Model file for the job. Use its own axes, mm. A direction names the side the tool comes from. Give positions to 0.01 mm unless a question says otherwise; leave off trailing zeros. Loops run counter-clockwise (first coordinate to the right, second up) from the corner with the lowest first, then second, coordinate; pieces in that order, holes last. Notation, with made-up numbers: M 33.5,27 L 37.5,27 A27 cw 37.5,59 Z; hole C -26,57 d10. An arc over 180 degrees is marked long. Answer in a Markdown table with one row per item.
```python
from build123d import *

# Parameters (mm, degrees)
SKETCH2_OUTSIDE_W       = 34.798
SKETCH2_OUTSIDE_H       = 34.798
CUT_EXTRUDE1_DEPTH      = 21.32
CUT_EXTRUDE1_DEPTH_BACK = 27.67
SKETCH3_R               = 5.55625
CUT_EXTRUDE2_DEPTH      = 20.05


with BuildPart() as part:
    # Sketch1 → Revolve1 (revolve)
    with BuildSketch(Plane.XY):
        Polygon((0, 10.795), (-7.62, 10.795), (-7.62, 7.747), (-27.94, 7.747), (-27.94, 0), (19.05, 0), (19.05, 5.55625), (0, 5.55625), align=None)
    revolve(axis=Axis((-27.94, 0, 0), (1, 0, 0)))

    # Sketch2 outside → Cut-Extrude1 (cut, two sides)
    with BuildSketch(Plane.ZY.offset(7.62)) as cut_extrude1_sk:
        Rectangle(SKETCH2_OUTSIDE_W, SKETCH2_OUTSIDE_H)
        Polygon((-5.499261314, 9.525), (-10.998522628, 0), (-5.499261314, -9.525), (5.499261314, -9.525), (10.998522628, 0), (5.499261314, 9.525), align=None, mode=Mode.SUBTRACT)
    extrude(amount=CUT_EXTRUDE1_DEPTH, mode=Mode.SUBTRACT)
    extrude(cut_extrude1_sk.sketch, amount=-CUT_EXTRUDE1_DEPTH_BACK, mode=Mode.SUBTRACT)

    # Sketch3 → Cut-Extrude2 (cut, through all)
    with BuildSketch(Plane(origin=(0, 0, 0), x_dir=(0, 0, -1), z_dir=(1, 0, 0))):
        Circle(SKETCH3_R)
    extrude(amount=CUT_EXTRUDE2_DEPTH, mode=Mode.SUBTRACT)


solid = part.part
```
Q1. Saw through at A-A (x = -4.5). Give the cut face in (y, z) (3 decimals), and give its area (3 significant figures).
Reported:
| item | result |
|---|---|
| outline | M -9.525,-5.08 A10.795 ccw -9.162,-5.709 L -0.363,-10.789 A10.795 ccw 0.363,-10.789 L 9.162,-5.709 A10.795 ccw 9.525,-5.08 L 9.525,5.08 A10.795 ccw 9.162,5.709 L 0.363,10.789 A10.795 ccw -0.363,10.789 L -9.162,5.709 A10.795 ccw -9.525,5.08 Z |
| area | 314 mm² |
Q2. Probe probe 1 along X at (y, z) = (7.25, 4); probe 2 along Z at (x, y) = (-5.25, 4); probe 3 along Y at (x, z) = (-9.5, 0.5). List the from-to ranges inside material, lowest first.
Reported:
| item | result |
|---|---|
| probe 1 | -7.62 to 0 |
| probe 2 | -8.69 to 8.69 |
| probe 3 | -7.73 to 7.73 |
Q3. Drop flat-ended pins along their axis: pin 1 (1.5 mm diameter, centred on x = -6.5, z = 7.5, fed in from -Y); pin 2 (1.5 mm diameter, centred on x = -14, z = -1.5, fed in from -Y); pin 3 (3 mm diameter, centred on x = -5.5, y = 2.5, fed in from +Z). Give the stop position or say it passes through.
Reported:
| item | result |
|---|---|
| pin 1 | y = -7.36 |
| pin 2 | y = -7.71 |
| pin 3 | z = 10.42 |
Q4. Saw through at D-D (x = -21.5). Give the cut face in (y, z), and give its area (3 significant figures).
Reported:
| item | result |
|---|---|
| outline | C 0,0 d15.49 |
| area | 189 mm² |
Q5. Saw through at C-C (y = 0). Give the cut face in (x, z) (3 decimals).
Reported:
| item | result |
|---|---|
| outline | M -27.94,-7.747 L -7.62,-7.747 L -7.62,-10.795 L 0,-10.795 L 0,10.795 L -7.62,10.795 L -7.62,7.747 L -27.94,7.747 Z |
Q6. 3-axis set-ups, long thin cutter, end or side, ignore diameter. For faces 1 (the face through (-7.62, -8, 1)), 2 (the face through (-4, -9.525, 0)): which of +Z, -Z, +X, -X, +Y, -Y reach the whole face in a straight line?
Reported:
| item | result |
|---|---|
| face 1 | -X |
| face 2 | +Z, -Z, +X, -X, -Y |
Q7. Saw through at B-B (z = 0). Give the cut face in (x, y) (3 decimals), and give its area (3 significant figures).
Reported:
| item | result |
|---|---|
| outline | M -27.94,-7.747 L -7.62,-7.747 L -7.62,-9.525 L 0,-9.525 L 0,9.525 L -7.62,9.525 L -7.62,7.747 L -27.94,7.747 Z |
| area | 460 mm² |
